Can you work these out from the drawing? Everything is in mm from the part's minimum corner. A direction names the side the tool comes from. Give positions to 0.01 mm unless a question says otherwise; leave off trailing zeros. Write each loop counter-clockwise with the first axis right and the second up, starting at its lowest first coordinate (ties: lowest second). Pieces come first, ordered by that corner, then holes. Notation, with made-up numbers: (-36.5, -35) -> (-19.5, -35) arc R23 cw to (-19.5, -26) -> close; hole circle Ø11 at (12, 70.5). An arc over 180 degrees is marked (long way). Write item = value, one per line. Start each with the question number.
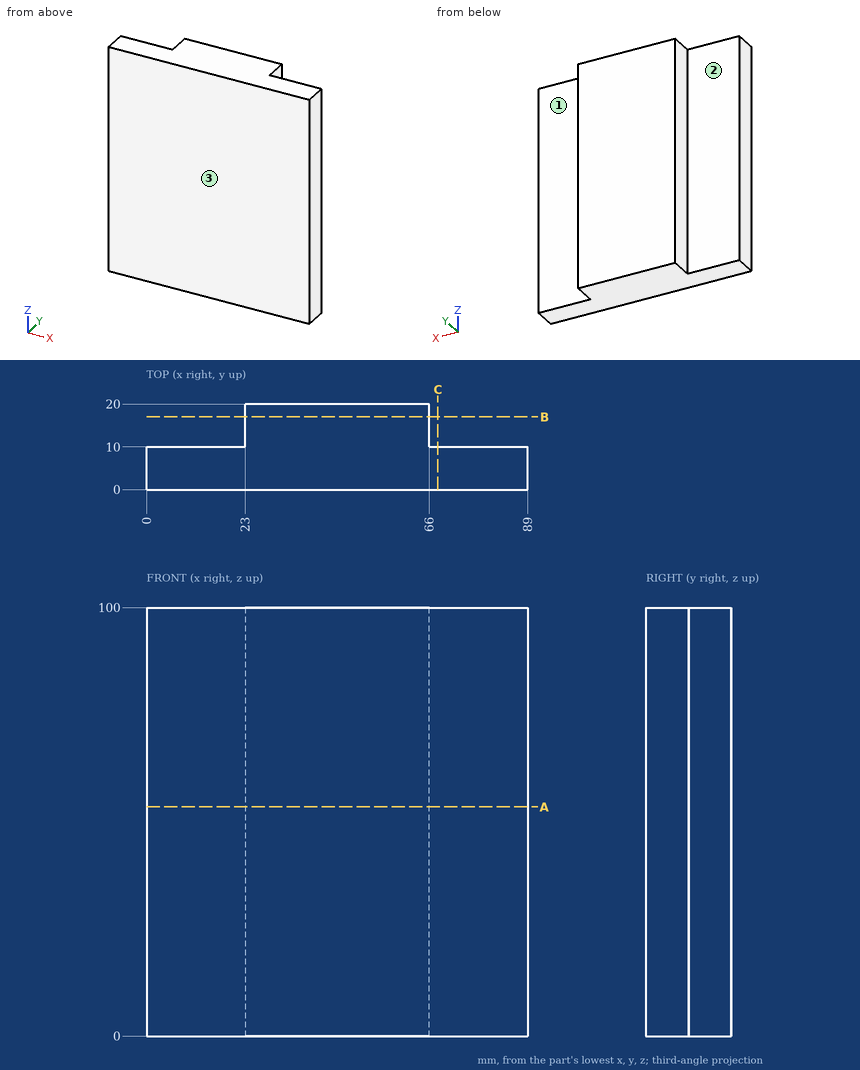
(1) Imagine slicing it at C-C (x = 68). Please give me the cut outline in (y, z).
(2) Imagine slicing it at B-B (y = 17). Please give me the cut outline in (x, z).
(3) On a 3-axis mill with a long thin cutter (end or side, diameter ignored), from which of +Z, -Z, +X, -X, +Y, -Y can I reach the whole of each face in a straight line? I mean the marked faces 1, 2 and 3. Say none if no direction works.
(4) Imagine slicing it at A-A (z = 53.5). Please give me the cut outline in (x, y), then the cut area to 3 significant figures.
(5) If I drill on line 1 along X through (y, z) = (14, 94); line 2 along Y through (x, z) = (83, 55), over which ranges is the centre line in solid material (lowest first)? Write a range as from..to.
(6) I'm going to push flat-ended pins straight in: pin 1 (11 mm diameter, centred on y = 16.5, z = 68.5, fed in from +X); pin 2 (8 mm diameter, centred on y = 14.5, z = 45.5, fed in from -X); pin 3 (18.5 mm diameter, centred on x = 7.5, z = 65, fed in from +Y). Where does each tip first touch, or does it pass through?
Answers below:
q1.outline = (0, 0) -> (10, 0) -> (10, 100) -> (0, 100) -> close
q2.outline = (23, 0) -> (66, 0) -> (66, 100) -> (23, 100) -> close
q3.face_1 = +Z, -Z, +X, +Y
q3.face_2 = +Z, -Z, -X, +Y
q3.face_3 = +Z, -Z, +X, -X, -Y
q4.outline = (0, 0) -> (89, 0) -> (89, 10) -> (66, 10) -> (66, 20) -> (23, 20) -> (23, 10) -> (0, 10) -> close
q4.area = 1,320 mm^2
q5.line_1 = 23..66
q5.line_2 = 0..10
q6.pin_1 = 66
q6.pin_2 = 23
q6.pin_3 = 10
